Could you check a few things on this model? Use its own coordinates, in mm. Face numbers are marked on the shaded views. Round coordinates to 2 decimals unless told otherwise and drop trailing zeros. Loops run counter-clockwise (first coordinate to the right, second up) from the corner with the lowest first, then second, coordinate; pieces in that order, holes last. Notation, with made-up numbers: M 75.5,59.25 L 104.5,59.25 A23 cw 104.5,78.25 Z; hole C 50.25,14.25 d4. An arc over 180 degrees is marked long. One line per item, written item: value. Start each with the question number.
Q1. Imagine slicing it at A-A (x = 0). Please give me the cut outline in (y, z).
Q2. I'm going to push flat-ended pins straight in: pin 1 Ø1.5 at (x, y) = (23, 11.5) entering from +Z; pin 2 Ø3.5 at (x, z) = (-36.5, -2) entering from +Y; pin 3 Ø5 at (x, z) = (51, 0) entering from -Y; pin 4 Ø1.5 at (x, y) = (28, 3) entering from -Z. Where does each tip first touch, or does it pass through?
Q3. Imagine slicing it at C-C (y = 11.75). Please give me the cut outline in (x, z), then the cut area to 3 significant figures.
Q4. Imagine slicing it at D-D (x = -49.5). Please give me the cut outline in (y, z), then the cut area to 3 significant figures.
Q5. Please list where these lines run through material, in increasing order: line 1 along X through (y, z) = (11.5, -10); line 2 along Z through (x, y) = (4.5, 3); line 3 along X through (y, z) = (13.25, 9).
Q6. Thinking about a two-plate mould opening in Z: for the marked faces 1, 2 and 3, which applies, released by +Z, released by -Z, zero draft, split by the parting line, or undercut?
Q7. Imagine slicing it at B-B (y = 5.5). Please give me the cut outline in (x, z), then the cut area to 3 significant figures.
from build123d import *

# Parameters (mm, degrees)
F0_R        = 3.25
F0_R_2      = 41.5
F0_R_3      = 2.75
F1_DEPTH    = 10
F2_DEPTH    = 15
F3_R        = 2.75
F4_DEPTH    = 12
F5_T2_ANGLE = 170.4527374882
F5_T4_ANGLE = 170.4527374882


# Not quite as in the source:
# - a fillet or chamfer that OpenCascade refuses, or shapes differently, is made with other operations: its cross-section is extruded or revolved along the edge and cut away or added


with BuildPart() as f1:
    # F0 (on Front) → F1 (new body)
    with BuildSketch(Plane.XZ):
        with BuildLine():
            Line((56.1470588235, 4.7442370796), (32.7205882353, 30.159792863))
            ThreePointArc((32.7205882353, 30.159792863), (0, 44.5), (-32.7205882353, 30.159792863))
            Line((-32.7205882353, 30.159792863), (-56.1470588235, 4.7442370796))
            ThreePointArc((-56.1470588235, 4.7442370796), (-58, 0), (-56.1470588235, -4.7442370796))
            Line((-56.1470588235, -4.7442370796), (-32.7205882353, -30.159792863))
            ThreePointArc((-32.7205882353, -30.159792863), (0, -44.5), (32.7205882353, -30.159792863))
            Line((32.7205882353, -30.159792863), (56.1470588235, -4.7442370796))
            ThreePointArc((56.1470588235, -4.7442370796), (58, 0), (56.1470588235, 4.7442370796))
        make_face()
        with Locations((-51, 0)):
            Circle(F0_R, mode=Mode.SUBTRACT)
        Circle(F0_R_2, mode=Mode.SUBTRACT)
        with Locations((51, 0)):
            Circle(F0_R, mode=Mode.SUBTRACT)
        Circle(F0_R_2)
        with BuildLine():
            ThreePointArc((-5.5275883623, 13.9443811945), (14.9403084329, -1.336855987), (-7.9154361587, -12.7415018902))
            Line((-7.9154361587, -12.7415018902), (-11.2935258895, -16.2148281895))
            ThreePointArc((-11.2935258895, -16.2148281895), (-16.2431437728, -16.28328537), (-16.3109133443, -11.3336580242))
            Line((-16.3109133443, -11.3336580242), (-12.8354378119, -7.7621863014))
            ThreePointArc((-12.8354378119, -7.7621863014), (-14.9994558699, -0.1277638746), (-12.9658008757, 7.5424139141))
            ThreePointArc((-12.9658008757, 7.5424139141), (-12.8781036996, 7.6911926971), (-12.7886994065, 7.8389519382))
            Line((-12.7886994065, 7.8389519382), (-16.1911722961, 11.1499710909))
            ThreePointArc((-16.1911722961, 11.1499710909), (-16.3869084591, 16.1374875976), (-11.3967981993, 16.2489916113))
            Line((-11.3967981993, 16.2489916113), (-7.8389519382, 12.7886994065))
            ThreePointArc((-7.8389519382, 12.7886994065), (-6.7082039325, 13.416407865), (-5.5275883623, 13.9443811945))
        make_face(mode=Mode.SUBTRACT)
        with Locations((-37.5, 0)):
            Circle(F0_R_3, mode=Mode.SUBTRACT)
        with Locations((37.5, 0)):
            Circle(F0_R_3, mode=Mode.SUBTRACT)
    extrude(amount=-F1_DEPTH)

    # F0 (on Front) → F2 (join)
    with BuildSketch(Plane.XZ):
        Circle(F0_R_2)
        with BuildLine():
            ThreePointArc((-5.5275883623, 13.9443811945), (14.9403084329, -1.336855987), (-7.9154361587, -12.7415018902))
            Line((-7.9154361587, -12.7415018902), (-11.2935258895, -16.2148281895))
            ThreePointArc((-11.2935258895, -16.2148281895), (-16.2431437728, -16.28328537), (-16.3109133443, -11.3336580242))
            Line((-16.3109133443, -11.3336580242), (-12.8354378119, -7.7621863014))
            ThreePointArc((-12.8354378119, -7.7621863014), (-14.9994558699, -0.1277638746), (-12.9658008757, 7.5424139141))
            ThreePointArc((-12.9658008757, 7.5424139141), (-12.8781036996, 7.6911926971), (-12.7886994065, 7.8389519382))
            Line((-12.7886994065, 7.8389519382), (-16.1911722961, 11.1499710909))
            ThreePointArc((-16.1911722961, 11.1499710909), (-16.3869084591, 16.1374875976), (-11.3967981993, 16.2489916113))
            Line((-11.3967981993, 16.2489916113), (-7.8389519382, 12.7886994065))
            ThreePointArc((-7.8389519382, 12.7886994065), (-6.7082039325, 13.416407865), (-5.5275883623, 13.9443811945))
        make_face(mode=Mode.SUBTRACT)
        with Locations((-37.5, 0)):
            Circle(F0_R_3, mode=Mode.SUBTRACT)
        with Locations((37.5, 0)):
            Circle(F0_R_3, mode=Mode.SUBTRACT)
    extrude(amount=-F2_DEPTH)

    # F3 (on face) → F4 (cut)
    with BuildSketch(Plane(origin=(0, 15, 0), x_dir=(-1, 0, 0), z_dir=(0, 1, 0))):
        with BuildLine():
            ThreePointArc((41.31, -3.9665980386), (42.5598913032, -2.1558061137), (43, 0))
            ThreePointArc((43, 0), (42.5598913032, 2.1558061137), (41.31, 3.9665980386))
            ThreePointArc((41.31, 3.9665980386), (41.4524727851, 1.9855729652), (41.5, 0))
            ThreePointArc((41.5, 0), (41.4524727851, -1.9855729652), (41.31, -3.9665980386))
        make_face()
        with BuildLine():
            ThreePointArc((41.5, 0), (41.4524727851, 1.9855729652), (41.31, 3.9665980386))
            ThreePointArc((41.31, 3.9665980386), (32, 0), (41.31, -3.9665980386))
            ThreePointArc((41.31, -3.9665980386), (41.4524727851, -1.9855729652), (41.5, 0))
        make_face()
        with Locations((37.5, 0)):
            Circle(F3_R, mode=Mode.SUBTRACT)
        with BuildLine():
            ThreePointArc((-41.31, -3.9665980386), (-41.5, 0), (-41.31, 3.9665980386))
            ThreePointArc((-41.31, 3.9665980386), (-43, 0), (-41.31, -3.9665980386))
        make_face()
        with BuildLine():
            ThreePointArc((-32, 0), (-35.3441938863, 5.0598913032), (-41.31, 3.9665980386))
            ThreePointArc((-41.31, 3.9665980386), (-41.5, 0), (-41.31, -3.9665980386))
            ThreePointArc((-41.31, -3.9665980386), (-35.3441938863, -5.0598913032), (-32, 0))
        make_face()
        with Locations((-37.5, 0)):
            Circle(F3_R, mode=Mode.SUBTRACT)
        with Locations((37.5, 0)):
            Circle(F3_R)
        with Locations((-37.5, 0)):
            Circle(F3_R)
    extrude(amount=-F4_DEPTH, mode=Mode.SUBTRACT)

    # F5: chamfer of 0.2 on 2 edges, made by hand

    # F5_s1 → F5_t2 (revolve, cut)
    with BuildSketch(Plane(origin=(0, 0, 0), x_dir=(0, 1, 0), z_dir=(0.0832192271, 0, -0.9965312641))):
        Polygon((14.8, 41.5), (15, 41.3), (15, 41.5), align=None)
    revolve(axis=Axis((0, 15, 0), (0, -1, 0)), revolution_arc=F5_T2_ANGLE, mode=Mode.SUBTRACT)

    # F5_s3 → F5_t4 (revolve, cut)
    with BuildSketch(Plane(origin=(0, 0, 0), x_dir=(0, 1, 0), z_dir=(-0.0832192271, 0, 0.9965312641))):
        Polygon((14.8, 41.5), (15, 41.3), (15, 41.5), align=None)
    revolve(axis=Axis((0, 15, 0), (0, -1, 0)), revolution_arc=F5_T4_ANGLE, mode=Mode.SUBTRACT)


solid = f1.part
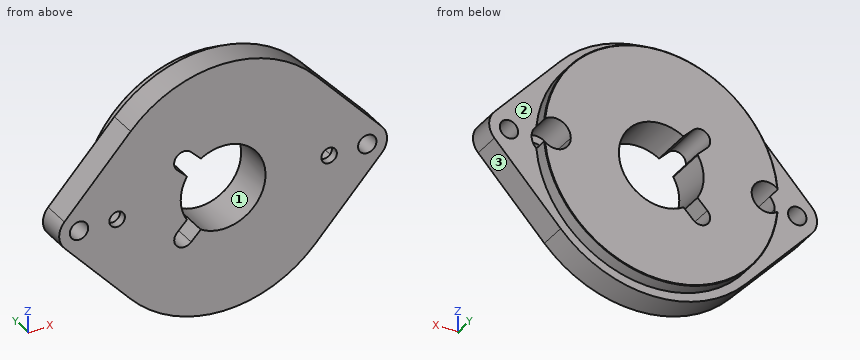
Report:
1. outline: M 0,-44.5 L 10,-44.5 L 10,-41.5 L 14.8,-41.5 L 15,-41.3 L 15,-15 L 0,-15 Z; M 0,15 L 15,15 L 15,41.3 L 14.8,41.5 L 10,41.5 L 10,44.5 L 0,44.5 Z
2. pin 1: stops at z = 35.03
2. pin 2: stops at y = 3
2. pin 3: passes through
2. pin 4: stops at z = -35.18
3. outline: M -41.31,-3.97 A41.5 ccw 41.31,-3.97 A5.5 cw long 41.31,3.97 A41.5 ccw -41.31,3.97 A5.5 cw long Z; hole M -16.31,-11.33 A3.5 ccw -11.29,-16.21 L -7.92,-12.74 A15 ccw long -7.84,12.79 L -11.4,16.25 A3.5 ccw long -16.19,11.15 L -12.79,7.84 A15 ccw -12.97,7.54 A15 ccw -12.84,-7.76 Z
3. area: 4,430 mm²
4. outline: M 0,-11.96 L 10,-11.96 L 10,-2.88 L 0,-2.88 Z; M 0,2.88 L 10,2.88 L 10,11.96 L 0,11.96 Z
4. area: 181 mm²
5. line 1: x = -40.28 to -15.01, 11.18 to 40.28
5. line 2: z = -44.27 to -14.31, 14.31 to 44.27
5. line 3: x = -40.51 to -13.98, 12 to 40.51
6. face 1: undercut
6. face 2: zero draft
6. face 3: released by -Z
7. outline: M -56.15,-4.74 L -32.72,-30.16 A44.5 ccw 32.72,-30.16 L 56.15,-4.74 A7 ccw 56.15,4.74 L 32.72,30.16 A44.5 ccw -32.72,30.16 L -56.15,4.74 A7 ccw Z; hole C -51,0 d6.5; hole C -37.5,0 d11; hole M -16.31,-11.33 A3.5 ccw -11.29,-16.21 L -7.92,-12.74 A15 ccw long -7.84,12.79 L -11.4,16.25 A3.5 ccw long -16.19,11.15 L -12.79,7.84 A15 ccw -12.97,7.54 A15 ccw -12.84,-7.76 Z; hole C 37.5,0 d11; hole C 51,0 d6.5
7. area: 5,840 mm²
